Verification items for the finished model (mm, model axes). A direction names the side the tool comes from. Round coordinates to 2 decimals unless told otherwise and drop trailing zeros. Write each loop counter-clockwise with the first axis right and the second up, starting at its lowest first coordinate (ties: lowest second). Pieces come first, ordered by that corner, then holes. Notation, with made-up numbers: M 68.25,72.5 L 77.25,72.5 A21 cw 77.25,111.5 Z; hole C 70.25,-3.75 d8. An arc over 180 degrees is marked long. Answer in a Markdown table with one row per item. Add a question column.
1. Sectioned sample at D-D on z = 19. Record the cut outline in (x, y), plus the area to 3 significant figures.
2. Set-up check for faces 4 (the flat face through (-31.25, -0.552, 16.825)), 5 (the flat face through (0, 0, 0)): record each of +Z, -Z, +X, -X, +Y, -Y from which the full face is reachable in a straight line by a thin tool's end or side.
3. Draft check along X on faces 1 (the flat face through (-0.59, 33.54, 14.79)), 2 (the flat face through (0, 0, 3)), 3 (the flat face through (-46.667, -0.716, 54.65)). Enter one of: pulls with the +X half, pulls with the -X half, needs draft (parallel to the pull), parting line crosses it, or undercut.
4. Sectioned sample at B-B on z = 36.5. Record the cut outline in (x, y), plus the area to 3 significant figures.
5. Material ranges on probe 1 along Y at (x, z) = (-18.5, 38.5); probe 2 along Y at (x, z) = (-14, 20); probe 3 along X at (y, z) = (-34, 63.5), recorded low to high.
6. Sectioned sample at A-A on y = -3.5. Record the cut outline in (x, z).
7. Go/stop test with flat-tipped pins: pin 1 Ø8 at (x, z) = (22, 17.5) entering from -Y; pin 2 Ø5 at (y, z) = (34, 50) entering from +X; pin 3 Ø3 at (x, y) = (37, 36) entering from +Z. Record where each tip stops, or that it passes through.
Autodesk Fusion 360 part; units mm, degrees
sketch "스케치1" plane through (0, 0, 0) normal (0, 0, 1) x (1, 0, 0)
  line L0 (-25, 25) -> (25, 25)
  line L1 (25, 25) -> (25, -25)
  line L2 (25, -25) -> (-25, -25)
  line L3 (-25, -25) -> (-25, 25)
extrude "돌출1" add sketch "스케치1" along normal blind 30 draft 30
extrude "돌출2" add 1 faces at (-14.1068, -14.1068, 30) along direction (0, 0, 1) blind 50 draft 10
shell "쉘1" thickness 3 removed faces 1 at (-17.0456, 17.0456, 80)
Geometry check:
| question | item | result |
|---|---|---|
| 1 | outline | M -35.97,-35.97 L 35.97,-35.97 L 35.97,35.97 L -35.97,35.97 Z; hole M -32.51,-32.51 L 32.51,-32.51 L 32.51,32.51 L -32.51,32.51 Z |
| 1 | area | 949 mm2 |
| 2 | face 4 | +Z |
| 2 | face 5 | -Z, +X, -X, +Y, -Y |
| 3 | face 1 | needs draft |
| 3 | face 2 | undercut |
| 3 | face 3 | pulls with the -X half |
| 4 | outline | M -43.47,-43.47 L 43.47,-43.47 L 43.47,43.47 L -43.47,43.47 Z; hole M -40.42,-40.42 L 40.42,-40.42 L 40.42,40.42 L -40.42,40.42 Z |
| 4 | area | 1,020 mm2 |
| 5 | probe 1 | y = -43.82 to -40.77, 40.77 to 43.82 |
| 5 | probe 2 | y = -36.55 to -33.08, 33.08 to 36.55 |
| 5 | probe 3 | x = -48.23 to -45.18, 45.18 to 48.23 |
| 6 | outline | M -51.14,80 L -42.32,30 L -25,0 L 25,0 L 42.32,30 L 51.14,80 L 48.09,80 L 39.46,31.04 L 23.27,3 L -23.27,3 L -39.46,31.04 L -48.09,80 Z |
| 7 | pin 1 | stops at y = -37.41 |
| 7 | pin 2 | stops at x = 46.29 |
| 7 | pin 3 | stops at z = 29.38 |
